Source: CAD feature listing. Evaluate the final solid. Frame: model axes, mm. Round coordinates to 2 decimals unless told otherwise and drop trailing zeros. Loops run counter-clockwise (first coordinate to the right, second up) from the corner with the lowest first, then second, coordinate; pieces in that order, holes last.
Item 1: Ray query, L1, parallel to Y at x = -27.65, z = 15.75; L2, parallel to X at y = 22.75, z = 15.5; L3, parallel to Z at x = 2, y = 22.75. Return the intervals inside material, ascending.
Item 2: Section query A-A on x = 6. Return loops of the section in (y, z).
Item 3: First-contact query: P1, Ø0.9, axis at y = 22.5, z = -0.5, coming from the -X side; P2, Ø2.5, axis at y = 6, z = -15, coming from the -X side; P3, Ø2, axis at x = -21.5, z = 19, coming from the -Y side; P4, Ø2.5, axis at y = 22, z = -15.75, coming from the +X side. Flat tips, straight axial feed; report the tip coordinate or a pass-through.
```python
from build123d import *

# Parameters (mm, degrees)
SKETCH1_W           = 58
SKETCH1_H           = 47.5
BOSS_EXTRUDE1_DEPTH = 28
FILLET3_R           = 6
SKETCH2_R           = 1.5
CUT_EXTRUDE1_DEPTH  = 3
CUT_EXTRUDE2_START  = -29
SKETCH3_R           = 1.5
CUT_EXTRUDE2_DEPTH  = 3


with BuildPart() as part:
    # Sketch1 → Boss-Extrude1 (new body)
    with BuildSketch(Plane(origin=(0, 0, 0), x_dir=(1, 0, 0), z_dir=(0, 1, 0))):
        Rectangle(SKETCH1_W, SKETCH1_H)
    extrude(amount=BOSS_EXTRUDE1_DEPTH)

    # Fillet3
    fillet3_edges = [part.edges().sort_by_distance(p)[0] for p in [
        (0, 28, 23.75),
        (0, 0, 23.75),
        (0, 0, -23.75),
        (0, 28, -23.75),
    ]]
    fillet(fillet3_edges, radius=FILLET3_R)

    # Sketch2 → Cut-Extrude1 (cut)
    with BuildSketch(Plane(origin=(29, 0, 0), x_dir=(0, 0, -1), z_dir=(1, 0, 0))):
        with Locations((0, 6)):
            Circle(SKETCH2_R)
        with Locations((-15.75, 22)):
            Circle(SKETCH2_R)
        with Locations((15.75, 22)):
            Circle(SKETCH2_R)
    extrude(amount=-CUT_EXTRUDE1_DEPTH, mode=Mode.SUBTRACT)

    # Sketch3 → Cut-Extrude2 (cut)
    with BuildSketch(Plane(origin=(0, 0, 0), x_dir=(0, 0, -1), z_dir=(1, 0, 0)).offset(CUT_EXTRUDE2_START)):
        with Locations((0.107591006, 22)):
            Circle(SKETCH3_R)
        with Locations((-15.75, 6)):
            Circle(SKETCH3_R)
        with Locations((15.75, 6)):
            Circle(SKETCH3_R)
    extrude(amount=CUT_EXTRUDE2_DEPTH, mode=Mode.SUBTRACT)


solid = part.part
```
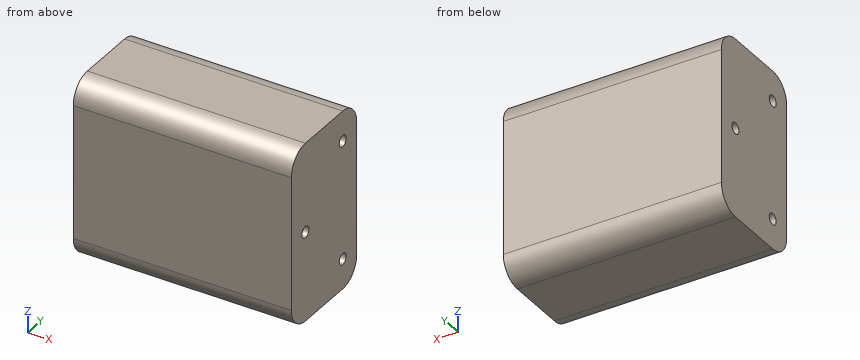
Data:
1. L1: y = 0 to 4.5, 7.5 to 28
1. L2: x = -29 to 26
1. L3: z = -23.7 to 23.7
2. outline: (0, -17.75) arc R6 ccw to (6, -23.75) - (22, -23.75) arc R6 ccw to (28, -17.75) - (28, 17.75) arc R6 ccw to (22, 23.75) - (6, 23.75) arc R6 ccw to (0, 17.75) - close
3. P1: stops at x = -26
3. P2: stops at x = -29
3. P3: stops at y = 0.01
3. P4: stops at x = 26
